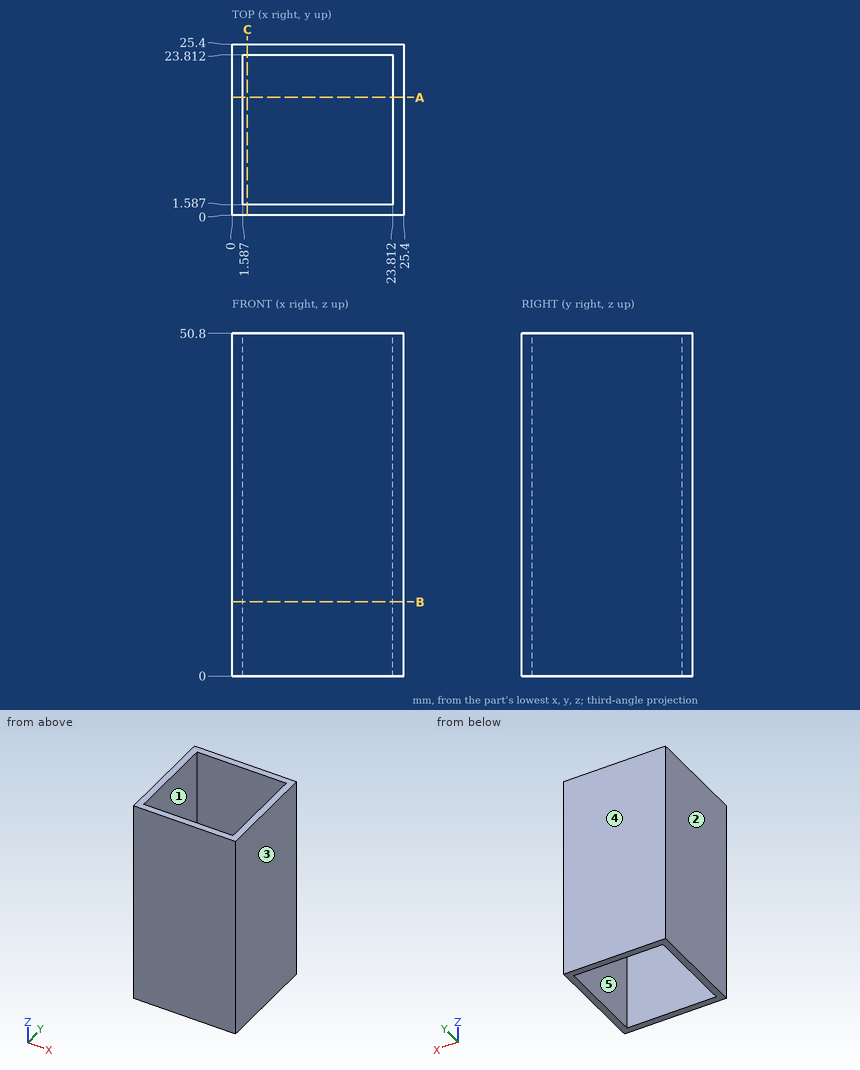
Part print with two shaded views. Sizes in mm from the minimum x, y, z corner. A direction names the side the tool comes from. Round coordinates to 2 decimals unless told otherwise and drop trailing zeros. Order: outer loops, then holes, each group sorted by start corner. A loop starts at its lowest first (then second) coordinate and runs counter-clockwise, first axis right, second up. Notation, with made-up numbers: (72.5, 63.25) - (82.5, 63.25) arc R37 cw to (82.5, 101.25) - close; hole circle Ø1 at (43, -3). An arc over 180 degrees is marked (long way). Return JSON: item names as keys, results as strings.
(1) Pull direction X, two halves, no side cores. Call the marked faces 1, 2 and 3: +X half, -X half, draft (parallel to the pull), parting line (faces both ways), or undercut.
Answer key:
{"face 1": "undercut", "face 2": "-X half", "face 3": "+X half"}
(2) Wall check: probe 1 along X at (y, z) = (18.75, 10.5). Give the ranges that are in metal, low to high. Write a range as from..to.
Answer key:
{"probe 1": "x = 0..1.59, 23.81..25.4"}
(3) Pin check, flat tips, straight feed: pin 1 Ø1.5 at (x, y) = (4, 14) entering from -Z; pin 2 Ø12 at (y, z) = (17.5, 11) entering from -X. Stop position of each tip, or through.
Answer key:
{"pin 1": "passes through", "pin 2": "stops at x = 0"}
(4) Cut at A-A (y = 17.5). Give the cut face in (x, z).
Answer key:
{"outline": "(0, 0) - (1.59, 0) - (1.59, 50.8) - (0, 50.8) - close; (23.81, 0) - (25.4, 0) - (25.4, 50.8) - (23.81, 50.8) - close"}
(5) Tool access for the marked faces 4 and 5: list every direction of +Z, -Z, +X, -X, +Y, -Y with a clear straight run to the whole face (end or side of a thin tool).
Answer key:
{"face 4": "+Z, -Z, +X, -X, +Y", "face 5": "+Z, -Z"}
(6) Cut at B-B (z = 11). Give the cut face in (x, y), then the cut area to 3 significant figures.
Answer key:
{"outline": "(0, 0) - (25.4, 0) - (25.4, 25.4) - (0, 25.4) - close; hole (1.59, 1.59) - (23.81, 1.59) - (23.81, 23.81) - (1.59, 23.81) - close", "area": "151 mm^2"}
